Here's the drawing with two shaded views (mm, measured from the low corner). I have some questions. A direction names the side the tool comes from. Coordinates: 2 decimals unless noted, no trailing zeros. Order: outer loops, then holes, each group sorted by start corner. A loop starts at its lowest first (then second) coordinate and runs counter-clockwise, first axis right, second up. Notation, with made-up numbers: (31, 8.5) -> (75, 8.5) arc R22 cw to (75, 15.5) -> close; hole circle Ø9 at (46, 18.5). An arc over 180 degrees is marked (long way). Return JSON: item names as keys, results as strings. Group by question number.
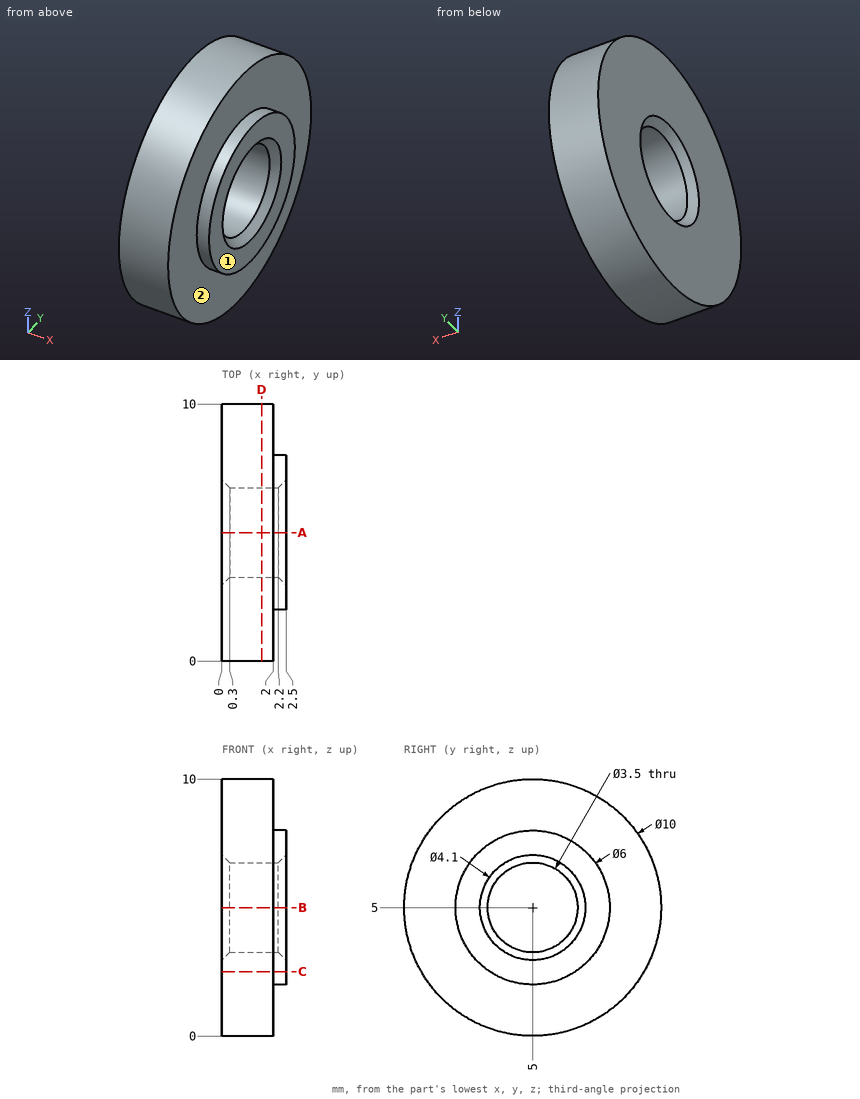
Q1. On a 3-axis mill with a long thin cutter (end or side, diameter ignored), from which of +Z, -Z, +X, -X, +Y, -Y can I reach the whole of each face in a straight line? I mean the marked faces 1 and 2. Say none if no direction works.
Q2. I need wall thicknesses on line 1 along Y through (x, z) = (1.1, 5); line 2 along X through (y, z) = (5.25, 9.25). Which ranges of each line are inside material? Lowest first, please. Write a range as from..to.
Q3. I want a section at C-C on z = 2.5. Please give me the cut outline in (x, y).
Q4. I want a section at A-A on y = 5. Please give me the cut outline in (x, z), and give its area (3 significant figures).
Q5. I want a section at D-D on x = 1.55. Please give me the cut outline in (y, z).
Q6. I'm going to push a flat-ended pin straight in: pin 1 Ø2 at (y, z) = (8.5, 2) entering from +X. Where does the tip first touch, or does it pass through?
Response values:
{
 "1": {"face 1": "+Z, -Z, +X, +Y, -Y", "face 2": "+X"},
 "2": {"line 1": "y = 0..3.25, 6.75..10", "line 2": "x = 0..2"},
 "3": {"outline": "(0, 0.67) -> (2, 0.67) -> (2, 3.34) -> (2.5, 3.34) -> (2.5, 6.66) -> (2, 6.66) -> (2, 9.33) -> (0, 9.33) -> close"},
 "4": {"outline": "(0, 0) -> (2, 0) -> (2, 2) -> (2.5, 2) -> (2.5, 2.95) -> (2.2, 3.25) -> (0.3, 3.25) -> (0, 2.95) -> close; (0, 7.05) -> (0.3, 6.75) -> (2.2, 6.75) -> (2.5, 7.05) -> (2.5, 8) -> (2, 8) -> (2, 10) -> (0, 10) -> close", "area": "14.1 mm²"},
 "5": {"outline": "circle Ø10 at (5, 5); hole circle Ø3.5 at (5, 5)"},
 "6": {"pin 1": "stops at x = 2"}
}
